For this review, take the finished solid that the model builds, in its own axes (mm). A direction names the side the tool comes from. Coordinates: 2 decimals unless noted, no trailing zeros. Order: outer loops, then holes, each group sorted by start corner. A loop starts at its lowest first (then second) coordinate and runs counter-clockwise, first axis right, second up. Notation, with made-up numbers: (38.5, -4.5) -> (48.5, -4.5) arc R18 ccw to (48.5, 24.5) -> close; hole circle Ø6 at (78.5, 55). An arc over 180 degrees is marked (long way). Answer as a JSON object with one key per item and string values. Group by question number.
1) Add section A-A, the plane y = 8. Write out the cut boundary in (x, z), then the cut area to 3 significant figures.
2) Add section D-D, the plane y = 1.5. Write out the cut boundary in (x, z).
3) For pin 1 (2 mm diameter, centred on x = 13.45, y = 2, fed in from -Z); pin 2 (1 mm diameter, centred on x = 2.5, z = 0.5, fed in from +Y); pin 3 (1 mm diameter, centred on y = 5, z = 0.5, fed in from +X), all flat-tipped, find the tip position at first contact; note any pin that passes through.
4) Add section B-B, the plane x = 3. Write out the cut boundary in (y, z).
5) Add section C-C, the plane z = 0.55. Write out the cut boundary in (x, y) (3 decimals), then the cut area to 3 significant figures.
6) Wall thickness on L1, parallel to X at y = 4.25, z = 0.3; L2, parallel to Y at x = 2.75, z = 1.1; L3, parallel to Y at x = 14.5, z = 1.8: over which ranges is each line inside the solid? List them lowest first.
7) Draft analysis for pull direction Y (two halves, no side actions). For faces 4 (the flat face through (8, 8, 0)), 5 (the cylindrical face through (2.2, 8.51, 0.99)), 6 (the flat face through (8, 0, 1)), state which applies: +Y half, -Y half, draft (parallel to the pull), parting line (faces both ways), or undercut.
8) Machinability: for faces 1 (the flat face through (12.2, 5, 1)), 2 (the flat face through (2, 4, 1)), 3 (the cylindrical face through (2.2, 2.51, 0.99)), which of the approach directions +Z, -Z, +X, -X, +Y, -Y give a long, thin tool a straight path to every point of the face, cutting with its end or side? Answer none if there is none.
from build123d import *

# Parameters (mm, degrees)
SKETCH2_R           = 0.75
SKETCH2_R_2         = 0.5
BOSS_EXTRUDE1_DEPTH = 2


with BuildPart() as part:
    # Sketch2 → Boss-Extrude1 (new body)
    with BuildSketch(Plane.XY):
        with BuildLine():
            Line((0, 9.945), (0, 6))
            Line((0, 6), (4, 6))
            Line((4, 6), (4, 4))
            Line((4, 4), (0, 4))
            Line((0, 4), (0, 2))
            ThreePointArc((0, 2), (0.585786438, 0.585786438), (2, 0))
            Line((2, 0), (14.2, 0))
            ThreePointArc((14.2, 0), (15.614213562, 0.585786438), (16.2, 2))
            Line((16.2, 2), (16.2, 4))
            Line((16.2, 4), (12.2, 4))
            Line((12.2, 4), (12.2, 6))
            Line((12.2, 6), (16.2, 6))
            Line((16.2, 6), (16.2, 9.945))
            ThreePointArc((16.2, 9.945), (14.735533906, 13.480533906), (11.2, 14.945))
            Line((11.2, 14.945), (5, 14.945))
            ThreePointArc((5, 14.945), (1.464466094, 13.480533906), (0, 9.945))
        make_face()
        with Locations((13.45, 8)):
            Circle(SKETCH2_R, mode=Mode.SUBTRACT)
        with Locations((13.45, 2)):
            Circle(SKETCH2_R, mode=Mode.SUBTRACT)
        with Locations((13.2, 11.942)):
            Circle(SKETCH2_R_2, mode=Mode.SUBTRACT)
        with Locations((3, 11.942)):
            Circle(SKETCH2_R_2, mode=Mode.SUBTRACT)
        with Locations((2.75, 2)):
            Circle(SKETCH2_R, mode=Mode.SUBTRACT)
        with Locations((2.75, 8)):
            Circle(SKETCH2_R, mode=Mode.SUBTRACT)
    extrude(amount=BOSS_EXTRUDE1_DEPTH)


solid = part.part
Output values:
{
 "1": {"outline": "(0, 0) -> (2, 0) -> (2, 2) -> (0, 2) -> close; (3.5, 0) -> (12.7, 0) -> (12.7, 2) -> (3.5, 2) -> close; (14.2, 0) -> (16.2, 0) -> (16.2, 2) -> (14.2, 2) -> close", "area": "26.4 mm²"},
 "2": {"outline": "(0.06, 0) -> (2.19, 0) -> (2.19, 2) -> (0.06, 2) -> close; (3.31, 0) -> (12.89, 0) -> (12.89, 2) -> (3.31, 2) -> close; (14.01, 0) -> (16.14, 0) -> (16.14, 2) -> (14.01, 2) -> close"},
 "3": {"pin 1": "stops at z = 0", "pin 2": "stops at y = 14.53", "pin 3": "stops at x = 12.2"},
 "4": {"outline": "(0, 0) -> (1.29, 0) -> (1.29, 2) -> (0, 2) -> close; (2.71, 0) -> (4, 0) -> (4, 2) -> (2.71, 2) -> close; (6, 0) -> (7.29, 0) -> (7.29, 2) -> (6, 2) -> close; (8.71, 0) -> (11.44, 0) -> (11.44, 2) -> (8.71, 2) -> close; (12.44, 0) -> (14.53, 0) -> (14.53, 2) -> (12.44, 2) -> close"},
 "5": {"outline": "(0, 2) arc R2 ccw to (2, 0) -> (14.2, 0) arc R2 ccw to (16.2, 2) -> (16.2, 4) -> (12.2, 4) -> (12.2, 6) -> (16.2, 6) -> (16.2, 9.945) arc R5 ccw to (11.2, 14.945) -> (5, 14.945) arc R5 ccw to (0, 9.945) -> (0, 6) -> (4, 6) -> (4, 4) -> (0, 4) -> close; hole circle Ø1.5 at (2.75, 2); hole circle Ø1.5 at (2.75, 8); hole circle Ø1 at (3, 11.942); hole circle Ø1.5 at (13.45, 2); hole circle Ø1.5 at (13.45, 8); hole circle Ø1 at (13.2, 11.942)", "area": "205 mm²"},
 "6": {"L1": "x = 4 to 12.2", "L2": "y = 0 to 1.25, 2.75 to 4, 6 to 7.25, 8.75 to 11.51, 12.38 to 14.41", "L3": "y = 0.02 to 4, 6 to 13.7"},
 "7": {"face 4": "draft", "face 5": "undercut", "face 6": "-Y half"},
 "8": {"face 1": "+Z, -Z, +X", "face 2": "+Z, -Z, -X", "face 3": "+Z, -Z"}
}
